Read the model definition and answer for the solid it produces. Units are mm, in the model's axes. A direction names the side the tool comes from. Coordinates: 2 decimals unless noted, no trailing zeros. Order: outer loops, then holes, each group sorted by start corner. A loop starts at its lowest first (then second) coordinate and runs counter-clockwise, first axis right, second up. Notation, with made-up numbers: (-34.5, -21.75) -> (16.5, -21.75) arc R5 cw to (16.5, -16.75) -> close; hole circle Ø6 at (11.25, -9.5). An arc over 180 degrees is marked (long way). Use CSV: the item, a comma, the result in double quotes.
```python
from build123d import *

# Parameters (mm, degrees)
SKETCH1_R                = 2.971068709
BOSS_EXTRUDE2_DEPTH      = 6
BOSS_EXTRUDE3_DEPTH      = 190
SKETCH3_R                = 2.971068709
BOSS_EXTRUDE5_DEPTH      = 6
SKETCH4_W                = 12.5
SKETCH4_H                = 10
BOSS_EXTRUDE6_DEPTH      = 11
SKETCH5_R                = 1
BOSS_EXTRUDE8_DEPTH      = 18
SKETCH5_2_R              = 1
CUT_EXTRUDE2_DEPTH       = 18
SKETCH7_R                = 6
SKETCH7_R_2              = 3.2
BOSS_EXTRUDE9_DEPTH      = 7.7
BOSS_EXTRUDE10_START     = -7.7
SKETCH8_R                = 6
SKETCH8_R_2              = 3.2
BOSS_EXTRUDE10_DEPTH     = 7.7
SKETCH9_W                = 182
SKETCH9_H                = 76.559305207
CUT_EXTRUDE3_DEPTH       = 6
SKETCH11_W               = 29
SKETCH11_H               = 25
CUT_EXTRUDE5_DEPTH       = 6
SKETCH12_W               = 29
SKETCH12_H               = 25
CUT_EXTRUDE6_DEPTH       = 6
SKETCH13_R               = 3.2
SKETCH13_R_2             = 3
CUT_EXTRUDE7_DEPTH       = 6
SKETCH14_R               = 3.2
CUT_EXTRUDE8_DEPTH       = 1273.798581799
SKETCH15_R               = 1
CUT_EXTRUDE9_DEPTH       = 11
SKETCH17_R               = 3
CUT_EXTRUDE11_DEPTH      = 170
CUT_EXTRUDE13_DEPTH      = 1271.151262578
CUT_EXTRUDE13_DEPTH_BACK = 1271.151262578
SKETCH19_R               = 3.2
SKETCH20_W               = 182
SKETCH20_H               = 76.559305207
CUT_EXTRUDE14_DEPTH      = 10


with BuildPart() as part:
    # Sketch1 → Boss-Extrude2 (new body)
    with BuildSketch(Plane(origin=(0, 0, 0), x_dir=(1, 0, 0), z_dir=(0, 1, 0))):
        Polygon((-40.573914373, 73.899203379), (-82.853566976, 0.668696943), (-40.573914373, -72.561809493), (43.985390835, -72.561809493), (86.265043438, 0.668696943), (43.985390835, 73.899203379), align=None)
        with Locations(Location((1.705738231, 0.668696943, 0), (0, 0, 270))):
            Circle(SKETCH1_R, mode=Mode.SUBTRACT)
    extrude(amount=BOSS_EXTRUDE2_DEPTH)

    # Sketch1<3> → Boss-Extrude3 (add)
    with BuildSketch(Plane(origin=(0, 0, 0), x_dir=(1, 0, 0), z_dir=(0, 1, 0))):
        Polygon((86.265043438, 0.668696943), (43.985390835, 73.899203379), (-40.573914373, 73.899203379), (-82.853566976, 0.668696943), (-40.573914373, -72.561809493), (43.985390835, -72.561809493), align=None)
        Polygon((-37.109812757, 67.899203379), (-75.925363746, 0.668696943), (-37.109812757, -66.561809493), (40.521289219, -66.561809493), (79.336840208, 0.668696943), (40.521289219, 67.899203379), align=None, mode=Mode.SUBTRACT)
    extrude(amount=BOSS_EXTRUDE3_DEPTH)

    # Sketch3 → Boss-Extrude5 (add)
    with BuildSketch(Plane(origin=(0, 190, 0), x_dir=(1, 0, 0), z_dir=(0, 1, 0))):
        Polygon((86.265043438, 0.668696943), (43.985390835, 73.899203379), (-40.573914373, 73.899203379), (-82.853566976, 0.668696943), (-40.573914373, -72.561809493), (43.985390835, -72.561809493), align=None)
        with Locations(Location((1.705738231, 0.668696943, 0), (0, 0, 270))):
            Circle(SKETCH3_R, mode=Mode.SUBTRACT)
    extrude(amount=BOSS_EXTRUDE5_DEPTH)

    # Sketch4 → Boss-Extrude6 (add)
    with BuildSketch(Plane(origin=(-62.429729502, 0, -36.043821133), x_dir=(-0.5000000000000001, 0, 0.8660254037844386), z_dir=(-0.8660254037844386, 0, -0.5000000000000001))):
        with Locations((2.755177243, 21.3)):
            Rectangle(SKETCH4_W, SKETCH4_H)
    extrude(amount=-BOSS_EXTRUDE6_DEPTH)

    # Sketch5 → Boss-Extrude8 (add)
    with BuildSketch(Plane.XZ):
        Polygon((40.521289219, -67.899203379), (11.391049027, -67.899203379), (11.391049027, -58.334458752), (46.043497104, -58.334458752), align=None)
        with Locations(Location((23.091264622, -63.273901871, 0), (0, 0, 270))):
            Circle(SKETCH5_R, mode=Mode.SUBTRACT)
    extrude(amount=-BOSS_EXTRUDE8_DEPTH)

    # Sketch5<2> → Cut-Extrude2 (cut)
    with BuildSketch(Plane.XZ):
        with Locations(Location((23.091264622, -63.273901871, 0), (0, 0, 270))):
            Circle(SKETCH5_2_R)
    extrude(amount=-CUT_EXTRUDE2_DEPTH, mode=Mode.SUBTRACT)

    # Sketch7 → Boss-Extrude9 (add)
    with BuildSketch(Plane(origin=(0, 196, 0), x_dir=(1, 0, 0), z_dir=(0, 1, 0))):
        with Locations(Location((1.705738231, 0.668696943, 0), (0, 0, 270))):
            Circle(SKETCH7_R)
        with Locations(Location((1.705738231, 0.668696943, 0), (0, 0, 270))):
            Circle(SKETCH7_R_2, mode=Mode.SUBTRACT)
    extrude(amount=-BOSS_EXTRUDE9_DEPTH)

    # Sketch8 → Boss-Extrude10 (add)
    with BuildSketch(Plane.XZ.offset(BOSS_EXTRUDE10_START)):
        with Locations(Location((1.705738231, -0.668696943, 0), (0, 0, 90))):
            Circle(SKETCH8_R)
        with Locations(Location((1.705738231, -0.668696943, 0), (0, 0, 90))):
            Circle(SKETCH8_R_2, mode=Mode.SUBTRACT)
    extrude(amount=BOSS_EXTRUDE10_DEPTH)

    # Sketch9 → Cut-Extrude3 (cut)
    with BuildSketch(Plane(origin=(629.826957164, 1366.496608068, -942.145548576), x_dir=(0, -1, 0), z_dir=(-0.8660254037844386, 0, -0.5000000000000003))):
        with Locations((1269.496608068, 1125.403480057)):
            Rectangle(SKETCH9_W, SKETCH9_H)
    extrude(amount=CUT_EXTRUDE3_DEPTH, mode=Mode.SUBTRACT)

    # Sketch11 → Cut-Extrude5 (cut)
    with BuildSketch(Plane(origin=(508.18415178, 1366.496608068, 1023.038661132), x_dir=(0, 1, 0), z_dir=(-0.8660254037844386, 0, 0.5000000000000001))):
        with Locations((-1345.996608068, 1169.575437511)):
            Rectangle(SKETCH11_W, SKETCH11_H)
    extrude(amount=-CUT_EXTRUDE5_DEPTH, mode=Mode.SUBTRACT)

    # Sketch12 → Cut-Extrude6 (cut)
    with BuildSketch(Plane(origin=(-287.090468893, 1366.496608068, 353.079993957), x_dir=(0, 1, 0), z_dir=(-0.8660254037844386, 0, -0.5000000000000001))):
        with Locations((-1345.996608068, 420.973803834)):
            Rectangle(SKETCH12_W, SKETCH12_H)
    extrude(amount=-CUT_EXTRUDE6_DEPTH, mode=Mode.SUBTRACT)

    # Sketch13 → Cut-Extrude7 (cut)
    with BuildSketch(Plane(origin=(690.748066702, 0, 917.635335707), x_dir=(-1, 0, 0), z_dir=(0, -1, 0))):
        with Locations(Location((754.924695238, 908.078431268, 0), (0, 0, 90))):
            Circle(SKETCH13_R)
        with Locations(Location((644.015452413, 885.008681135, 0), (0, 0, 90))):
            Circle(SKETCH13_R)
        with Locations(Location((642.689368477, 965.287041279, 0), (0, 0, 90))):
            Circle(SKETCH13_R_2)
    extrude(amount=-CUT_EXTRUDE7_DEPTH, mode=Mode.SUBTRACT)

    # Sketch14 → Cut-Extrude8 (cut, through all)
    with BuildSketch(Plane(origin=(690.748066702, 0, 917.635335707), x_dir=(-1, 0, 0), z_dir=(0, -1, 0))):
        with Locations(Location((644.015452413, 885.008681135, 0), (0, 0, 90))):
            Circle(SKETCH14_R)
    extrude(amount=-CUT_EXTRUDE8_DEPTH, mode=Mode.SUBTRACT)

    # Sketch15 → Cut-Extrude9 (cut)
    with BuildSketch(Plane(origin=(690.748066702, 16.3, 917.635335707), x_dir=(-1, 0, 0), z_dir=(0, -1, 0))):
        with Locations(Location((747.475715997, 946.555449467, 0), (0, 0, 90))):
            Circle(SKETCH15_R)
    extrude(amount=-CUT_EXTRUDE9_DEPTH, mode=Mode.SUBTRACT)

    # Sketch17 → Cut-Extrude11 (cut)
    with BuildSketch(Plane(origin=(690.748066702, 198, 917.635335707), x_dir=(1, 0, 0), z_dir=(0, 1, 0))):
        with Locations(Location((-754.924695238, 908.078431268, 0), (0, 0, 270))):
            Circle(SKETCH17_R)
    extrude(amount=-CUT_EXTRUDE11_DEPTH, mode=Mode.SUBTRACT)

    # Sketch19 → Cut-Extrude13 (cut, two sides: drawn at the far end of the back side and taken through both)
    with BuildSketch(Plane(origin=(690.748066702, 18, 917.635335707), x_dir=(-1, 0, 0), z_dir=(0, -1, 0)).offset(-CUT_EXTRUDE13_DEPTH_BACK)):
        with Locations(Location((754.924695238, 908.078431268, 0), (0, 0, 90))):
            Circle(SKETCH19_R)
    extrude(amount=CUT_EXTRUDE13_DEPTH + CUT_EXTRUDE13_DEPTH_BACK, mode=Mode.SUBTRACT)

    # Sketch20 → Cut-Extrude14 (cut)
    with BuildSketch(Plane(origin=(-165.447663504, 1366.496608068, -436.647894277), x_dir=(0, -1, 0), z_dir=(-0.8660254037844385, 0, 0.5000000000000002))):
        with Locations((1269.496608068, 465.14576128)):
            Rectangle(SKETCH20_W, SKETCH20_H)
    extrude(amount=CUT_EXTRUDE14_DEPTH, mode=Mode.SUBTRACT)


solid = part.part
```
Item 1: A tool of negligible diameter and unlimited length cuts with its end or side. For faces 4 (the flat face through (-55, 16.3, -29)), 5 (the flat face through (-1, 188.3, 2)), 6 (the flat face through (-67.79, 20.3, -20.84)), from which of +Z, -Z, +X, -X, +Y, -Y can it reach the whole face along a straight path? Write none if from no direction.
Return value:
face 4,"+X"
face 5,"none"
face 6,"-X"
Item 2: Each of these flat-tipped pins is pushed along its axis until it touches: P1, Ø1.9, axis at x = 3, z = -1, coming from the -Y side; P2, Ø7, axis at x = 2.5, z = -0.5, coming from the +Y side; P3, Ø7.5, axis at y = 12.5, z = -62.5, coming from the -X side; P4, Ø2, axis at y = 94.5, z = -57.5, coming from the +X side. Where does it stop, or does it pass through?
Return value:
P1,"passes through"
P2,"stops at y = 196"
P3,"stops at x = -49.32"
P4,"stops at x = -42.54"
Item 3: Find section C-C, the plane x = 71. Give the vertices of the cut face in (y, z).
Return value:
outline,"(0, -27.11) -> (6, -27.11) -> (6, 25.77) -> (0, 25.77) -> close; (188, -27.11) -> (196, -27.11) -> (196, 25.77) -> (188, 25.77) -> (188, 13.77) -> (190, 13.77) -> (190, -15.11) -> (188, -15.11) -> close"
Item 4: Straight lines are drawn through the part: line 1 along Y through (x, z) = (-53, 25.5); line 2 along Z through (x, y) = (27, 84); line 3 along Z through (x, y) = (-66, 16). For each, find the intervals that lie inside material, in ascending order.
Return value:
line 1,"y = 0 to 6, 190 to 196"
line 2,"z = -73.9 to -67.9, 66.56 to 72.56"
line 3,"z = -29.86 to -19.81, 18.47 to 28.52"
Item 5: The mould has two halves that part along Y. Classify faces 1 (the flat face through (-16, 0, 0)), 2 (the flat face through (-55, 26.3, -29)), 3 (the flat face through (47.802, 97.543, 65.952)): +Y half, -Y half, draft (parallel to the pull), parting line (faces both ways), or undercut.
Return value:
face 1,"-Y half"
face 2,"undercut"
face 3,"draft"
Item 6: Find section A-A, the plane x = -20.5. Give the vertices of the cut face in (y, z), then the cut area to 3 significant figures.
Return value:
outline,"(0, -73.9) -> (196, -73.9) -> (196, 72.56) -> (0, 72.56) -> close; hole (6, -67.9) -> (190, -67.9) -> (190, 66.56) -> (6, 66.56) -> close"
area,"3,970 mm^2"
Item 7: Find section B-B, the plane z = -16. Give the vertices of the cut face in (x, y), then the cut area to 3 significant figures.
Return value:
outline,"(-74, 0) -> (77.41, 0) -> (77.41, 6) -> (-74, 6) -> close; (-74, 35) -> (-67.07, 35) -> (-67.07, 190) -> (70.49, 190) -> (70.49, 188) -> (77.41, 188) -> (77.41, 196) -> (-74, 196) -> close"
area,"2,900 mm^2"
Item 8: Find section D-D, the plane y = 78.5. Give the vertices of the cut face in (x, z).
Return value:
outline,"(-82.85, -0.67) -> (-40.57, -73.9) -> (43.99, -73.9) -> (47.99, -66.97) -> (42.79, -63.97) -> (40.52, -67.9) -> (-37.11, -67.9) -> (-75.93, -0.67) -> (-37.11, 66.56) -> (40.52, 66.56) -> (42.79, 62.63) -> (47.99, 65.63) -> (43.99, 72.56) -> (-40.57, 72.56) -> close"
